The model under review builds one solid part; all positions refer to its coordinate system, in mm. Give positions to 0.01 mm unless a question says otherwise; leave off trailing zeros. Order: outer loops, then holes, each group sorted by start corner. A loop starts at its lowest first (then second) coordinate and runs counter-clockwise, first axis right, second up. Notation, with made-up numbers: (8.25, -21) - (13.25, -21) arc R22 cw to (13.25, 2) - close; hole circle Ø6 at (4, 53). An arc over 180 degrees is marked (long way). Use a Markdown table: item, result. Add a question column.
```python
from build123d import *

# Parameters (mm, degrees)
F2_W     = 5.461
F2_H     = 8.89
F3_DEPTH = 32.895429
F5_DEPTH = 32.895429
F7_DEPTH = 32.895429


with BuildPart() as f1:
    # F0 (on Top) → F1 (revolve)
    with BuildSketch(Plane.XY):
        with BuildLine():
            Line((0, 32.894429), (0, -32.894429))
            ThreePointArc((0, -32.894429), (32.894429, 0), (0, 32.894429))
        make_face()
    revolve(axis=Axis((0, 0, 0), (0, -1, 0)))

    # F2 (on Front) → F3 (cut, through all)
    with BuildSketch(Plane.XZ):
        with Locations((-10.487013, 11.237753)):
            Rectangle(F2_W, F2_H)
    extrude(amount=F3_DEPTH, mode=Mode.SUBTRACT)

    # F4 (on Front) → F5 (cut, through all)
    with BuildSketch(Plane.XZ):
        Polygon((11.933651, 15.546253), (6.895673, 15.557211), (6.895673, 6.736375), (11.933651, 6.736375), align=None)
    extrude(amount=F5_DEPTH, mode=Mode.SUBTRACT)

    # F6 (on Front) → F7 (cut, through all)
    with BuildSketch(Plane.XZ):
        Polygon((-10.553785, -7.94562), (-17.987287, -1.999777), (-21.413613, -6.356075), (-13.522841, -12.667675), (-4.894031, -15.459277), (7.455942, -15.459277), (15.173362, -12.460908), (20.658924, -8.790475), (17.52286, -4.103541), (11.391848, -8.20585), (4.74029, -10.79227), (-3.879014, -10.79227), align=None)
    extrude(amount=F7_DEPTH, mode=Mode.SUBTRACT)


solid = f1.part
```
Q1. We need section C-C (x = 9.5). Write out the cut boundary in (y, z), plus the area to 3 significant figures.
Q2. Clearance check with flat-ended pins moving along their axes: P1, Ø1.5, axis at y = 5.5, z = -19.5, coming from the +X side; P2, Ø6, axis at x = -18, z = 23.5, coming from the -Y side; P3, Ø1, axis at y = 20, z = -21.5, coming from the -X side. State where each tip first meets the part, or that it passes through.
Q3. Draft analysis for pull direction X (two halves, no side actions). For faces 1 (the flat face through (1, -14, -15.459)), 2 (the flat face through (6.896, -16, 11)), state which applies: pulls with the +X half, pulls with the -X half, needs draft (parallel to the pull), parting line crosses it, or undercut.
Q4. Wall thickness on probe 1 along Z at (x, y) = (-10.5, -7); probe 2 along Z at (x, y) = (-8, -10.5); probe 3 along X at (y, z) = (-14, -6): over which ranges is each line inside the solid? List them lowest first.
Q5. We need section D-D (y = -18). Write out the cut boundary in (x, z), plus the area to 3 significant figures.
Q6. We need section B-B (z = 13.5). Write out the cut boundary in (x, y), plus the area to 3 significant figures.
Q7. We need section A-A (y = -8). Write out the cut boundary in (x, z), plus the area to 3 significant figures.
Here are the results:
| question | item | result |
|---|---|---|
| 1 | outline | (-30.76, 6.74) arc R31.49 ccw to (-30.2, -8.94) - (0, -8.94) - (0, -14.67) - (-27.87, -14.67) arc R31.49 ccw (long way) to (-27.39, 15.55) - (0, 15.55) - (0, 6.74) - close |
| 1 | area | 2,690 mm2 |
| 2 | P1 | x = 26.48 |
| 2 | P2 | y = -19.35 |
| 2 | P3 | x = -15.78 |
| 3 | face 1 | undercut |
| 3 | face 2 | undercut |
| 4 | probe 1 | -30.38 to -13.65, -7.97 to 6.79, 15.68 to 30.38 |
| 4 | probe 2 | -30.13 to -14.45, -9.03 to 6.79, 15.68 to 30.13 |
| 4 | probe 3 | -29.16 to -21.13, -12.99 to 14.69, 18.79 to 29.16 |
| 5 | outline | circle Ø55.07 at (0, 0); hole (-21.41, -6.36) - (-13.52, -12.67) - (-4.89, -15.46) - (7.46, -15.46) - (15.17, -12.46) - (20.66, -8.79) - (17.52, -4.1) - (11.39, -8.21) - (4.74, -10.79) - (-3.88, -10.79) - (-10.55, -7.95) - (-17.99, -2) - close; hole (-13.22, 6.79) - (-7.76, 6.79) - (-7.76, 15.68) - (-13.22, 15.68) - close; hole (6.9, 6.74) - (11.93, 6.74) - (11.93, 15.55) - (6.9, 15.56) - close |
| 5 | area | 2,060 mm2 |
| 6 | outline | (-13.22, -26.93) - (-13.22, 0) - (-7.76, 0) - (-7.76, -28.98) arc R30 ccw to (6.9, -29.19) - (6.9, 0) - (11.93, 0) - (11.93, -27.52) arc R30 ccw (long way) to start |
| 6 | area | 2,530 mm2 |
| 7 | outline | circle Ø63.81 at (0, 0); hole (-21.41, -6.36) - (-13.52, -12.67) - (-4.89, -15.46) - (7.46, -15.46) - (15.17, -12.46) - (20.66, -8.79) - (17.52, -4.1) - (11.39, -8.21) - (4.74, -10.79) - (-3.88, -10.79) - (-10.55, -7.95) - (-17.99, -2) - close; hole (-13.22, 6.79) - (-7.76, 6.79) - (-7.76, 15.68) - (-13.22, 15.68) - close; hole (6.9, 6.74) - (11.93, 6.74) - (11.93, 15.55) - (6.9, 15.56) - close |
| 7 | area | 2,880 mm2 |
